from build123d import *

# Parameters (mm, degrees)
CUT_EXTRUDE1_REACH = 44.426
SKETCH2_R          = 5.05


with BuildPart() as part:
    # Sketch1 → Revolve1 (revolve)
    with BuildSketch(Plane.XY, mode=Mode.PRIVATE) as revolve1_sk:
        Polygon((0, 0), (10, 0), (10, 5), (7.5, 5), (7.5, 40), (0, 40), align=None)
    revolve(revolve1_sk.sketch.rotate(Axis((0, 45, 0), (0, -1, 0)), 180), axis=Axis((0, 45, 0), (0, -1, 0)))

    # Sketch2 → Cut-Extrude1 (cut, up to next)
    with BuildSketch(Plane(origin=(0, 40, 0), x_dir=(1, 0, 0), z_dir=(0, 1, 0)), mode=Mode.PRIVATE) as cut_extrude1_sk1:
        with Locations(Location((0, 0, 0), (0, 0, 270))):
            Circle(SKETCH2_R)
    cut_extrude1_tool1 = extrude(cut_extrude1_sk1.sketch, amount=-CUT_EXTRUDE1_REACH, mode=Mode.PRIVATE) & part.part
    add(cut_extrude1_tool1.solids().sort_by_distance((0, 40, 0))[0], mode=Mode.SUBTRACT)

    # Cut-Sweep1: sweep along a curve in space
    with BuildLine() as cut_sweep1_path:
        ThreePointArc((0, 40, 5.05), (3.570889245, 40, 3.570889245), (5.05, 40, 0))
        ThreePointArc((5.05, 40, 0), (3.570889245, 40, -3.570889245), (0, 40, -5.05))
        ThreePointArc((0, 40, -5.05), (-3.570889245, 40, -3.570889245), (-5.05, 40, 0))
        ThreePointArc((-5.05, 40, 0), (-3.570889245, 40, 3.570889245), (0, 40, 5.05))
    # Sketch3 → Cut-Sweep1 (sweep, cut)
    with BuildSketch(Plane.XY):
        Polygon((5.05, 36.8), (6.013641914, 0), (5.05, 0), align=None)
    sweep(path=cut_sweep1_path.line, mode=Mode.SUBTRACT)


solid = part.part
Can you work these out from the model? Positions are in its coordinate system, mm. A direction names the side the tool comes from. Round coordinates to 2 decimals unless told otherwise and drop trailing zeros. Loops run counter-clockwise (first coordinate to the right, second up) from the corner with the lowest first, then second, coordinate; pieces in that order, holes last. Notation, with made-up numbers: (-2.5, 75) - (34.5, 75) arc R25 cw to (34.5, 95) - close; hole circle Ø5 at (25, 16.5). An arc over 180 degrees is marked (long way). Write item = value, one per line. Start each with the question number.
(1) For faces 4 (the face through (-4.032, 22.745, -6.324)), 5 (the face through (0, 0, 7)), which set-ups out of +Z, -Z, +X, -X, +Y, -Y let a thin tool reach every point of the face, with its end or its side?
(2) If we section it at A-A (y = 25.5): Please give me the cut outline in (x, z), and give its area (3 significant figures).
(3) If we section it at C-C (y = 15): Please give me the cut outline in (x, z), and give its area (3 significant figures).
(4) For P1, Ø12, axis at x = -5, y = 24, coming from the -Z side; P2, Ø12, axis at y = 21, z = 4.5, coming from the -X side; P3, Ø1.5, axis at x = 7, y = 12.5, coming from the -Z side, each with a flat end and sliding along its axis, tell me the tip position at first contact or that it passes through.
(5) If I drill on probe 1 along X at (y, z) = (2, -4.5); probe 2 along Z at (x, y) = (5.25, 3); probe 3 along X at (y, z) = (3, -0.75), over which ranges is the centre line in solid material (lowest first)? Write a range as [from, to].
(6) If we section it at B-B (x = -7): Please give me the cut outline in (y, z), and give its area (3 significant figures).
(7) If we mould it in two halves opening along X, with no side actions, what happens to faces 1 (the face through (10, 3, 0)), 2 (the face through (1.517, 38.422, 4.817)), 3 (the face through (-4, 5, -7))? For each: released by +X, released by -X, zero draft, split by the parting line, or undercut.
Ans:
q1.face_4 = +Y
q1.face_5 = +Z, -Z, +X, -X, -Y
q2.outline = circle Ø15 at (0, 0); hole circle Ø10.69 at (0, 0)
q2.area = 86.9 mm²
q3.outline = circle Ø15 at (0, 0); hole circle Ø11.24 at (0, 0)
q3.area = 77.5 mm²
q4.P1 = -7.5
q4.P2 = -7.5
q4.P3 = -4.15
q5.probe_1 = [-8.93, -3.91], [3.91, 8.93]
q5.probe_2 = [-8.51, -2.77], [2.77, 8.51]
q5.probe_3 = [-9.97, -5.89], [5.89, 9.97]
q6.outline = (0, -7.14) - (5, -7.14) - (5, -2.69) - (40, -2.69) - (40, 2.69) - (5, 2.69) - (5, 7.14) - (0, 7.14) - close
q6.area = 260 mm²
q7.face_1 = split by the parting line
q7.face_2 = undercut
q7.face_3 = zero draft
